Can you work these out from the model? Positions are in its coordinate system, mm. Face numbers are marked on the shaded views. A direction names the side the tool comes from. Give positions to 0.01 mm unless a question says otherwise; leave off trailing zeros. Order: outer loops, then holes, each group sorted by start corner. A loop starts at its lowest first (then second) coordinate and runs counter-clockwise, first axis right, second up.
Item 1: I want a section at D-D, the plane y = -7.75. Write out the boundary of the cut face in (x, z).
Item 2: Which directions (+Z, -Z, +X, -X, +Y, -Y) give clear straight access to the entire face, cutting with the end or side of a thin tool? Please do the marked faces 5 and 6.
Item 3: I want a section at C-C, the plane x = 3.5. Write out the boundary of the cut face in (y, z), then the cut area to 3 significant figures.
Item 4: I'm going to push flat-ended pins straight in: pin 1 Ø1.5 at (x, z) = (-1.5, 2) entering from +Y; pin 2 Ø1.5 at (y, z) = (10, 2.5) entering from +X. Where does each tip first touch, or does it pass through?
Item 5: If I drill on line 1 along X through (y, z) = (1.75, 2.75); line 2 along Y through (x, z) = (0.25, 2.2); line 3 along X through (y, z) = (9.25, 1.2), over which ranges is the centre line in solid material (lowest first)?
Item 6: I want a section at B-B, the plane z = 0.75. Write out the boundary of the cut face in (x, y).
Item 7: I want a section at A-A, the plane y = 5. Write out the boundary of the cut face in (x, z).
Item 8: If we mould it in two halves opening along X, with no side actions, what happens to the marked faces 1, 2, 3 and 4? For each: +X half, -X half, draft (parallel to the pull), parting line (faces both ways), or undercut.
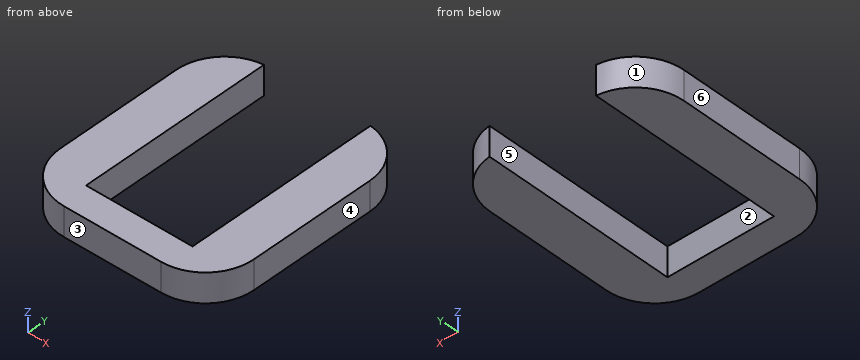
Autodesk Inventor part; units mm, degrees
ref_plane "YZ Plane" through (0, 0, 0) normal (1, 0, 0) x (0, 1, 0)
ref_plane "XZ Plane" through (0, 0, 0) normal (0, 1, 0) x (-1, 0, 0)
ref_plane "XY Plane" through (0, 0, 0) normal (0, 0, 1) x (1, 0, 0)
sketch "Boceto1" plane through (0, 0, 0) normal (0, 0, 1) x (1, 0, 0)
  line L0 (-10, -10) -> (10, -10)
  line L1 (10, -10) -> (10, 10)
  line L2 (-10, 10) -> (-10, -10)
  line L3 (-10, -10) -> (10, 10) construction
  line L4 (10, -10) -> (-10, 10) construction
  circle A0 centre (0, 0) radius 5.5
  line L5 (-5.5, 0) -> (-5.5, 11.2745)
  line L6 (-5.5, 11.2745) -> (-5.5, 10)
  line L7 (5.5, 0) -> (5.5, 6.4261)
  line L8 (5.5, 6.4261) -> (5.5, 10.6373)
  line L9 (-5.5, 0) -> (-5.5, -7)
  line L10 (-5.5, -7) -> (5.5, -7)
  line L11 (5.5, -7) -> (5.5, 0)
  line L12 (-5.5, 10) -> (-5.5, 13)
  line L13 (-5.5, 13) -> (-10, 13)
  line L14 (-10, 13) -> (-10, 10)
  line L15 (5.5, 10) -> (5.5, 13)
  line L16 (10, 13) -> (10, 10)
  line L17 (5.5, 13) -> (10, 13)
  dimension "d0" = 20
  dimension "d1" = 20
  dimension "d2" = 11
  dimension "d4" = 7
  dimension "d5" = 3
  dimension "d6" = 23
extrude "Extrusión1" add sketch "Boceto1" along normal blind 3 contours L2 L14 L13 L12 L5 L9 L10 L11 L7 L8 L15 L17 L16 L1 L0
fillet "Empalme1" radius 5 4 edges at (10, -10, 1.5) (-10, -10, 1.5) (-10, 13, 1.5) (10, 13, 1.5)
properties part number "seguro2"
Results list:
1. outline: (-9.18, 0) - (9.18, 0) - (9.18, 3) - (-9.18, 3) - close
2. face 5: +Z, -Z, +Y
2. face 6: +Z, -Z, -X, +Y, -Y
3. outline: (-10, 0) - (-7, 0) - (-7, 3) - (-10, 3) - close
3. area: 9.00 mm2
4. pin 1: stops at y = -7
4. pin 2: stops at x = 9.85
5. line 1: x = -10 to -5.5, 5.5 to 10
5. line 2: y = -10 to -7
5. line 3: x = -9.85 to -5.5, 5.5 to 9.85
6. outline: (-10, -5) arc R5 ccw to (-5, -10) - (5, -10) arc R5 ccw to (10, -5) - (10, 8.03) arc R5 ccw to (5.5, 13) - (5.5, -7) - (-5.5, -7) - (-5.5, 13) arc R5 ccw to (-10, 8.03) - close
7. outline: (-10, 0) - (-5.5, 0) - (-5.5, 3) - (-10, 3) - close; (5.5, 0) - (10, 0) - (10, 3) - (5.5, 3) - close
8. face 1: -X half
8. face 2: undercut
8. face 3: draft
8. face 4: +X half
